Work out the finished part from the listing and answer in its coordinate system (mm). Face numbers are marked on the shaded views. Give positions to 0.01 mm unless a question says otherwise; leave off trailing zeros. Order: outer loops, then holes, each group sorted by start corner. A loop starts at its lowest first (then second) coordinate and runs counter-clockwise, first axis right, second up. Notation, with made-up numbers: M -10.75,78 L 23.25,78 A33 cw 23.25,108 Z; hole C 31,-9.75 d7. An arc over 180 degrees is marked long. One line per item, written item: value.
from build123d import *

# Parameters (mm, degrees)
SKETCH1_W           = 12.7
SKETCH1_H           = 20.193
BOSS_EXTRUDE1_DEPTH = 6.35
SKETCH3_R           = 1.524
CUT_EXTRUDE1_DEPTH  = 25.685415715
SKETCH4_R           = 2.794
CUT_EXTRUDE2_DEPTH  = 0.762
SKETCH8_R           = 1.1938
CUT_EXTRUDE5_DEPTH  = 25.685415715
CUT_EXTRUDE7_DEPTH  = 25.685415715
CUT_EXTRUDE8_DEPTH  = 25.685415715


with BuildPart() as part:
    # Sketch1 → Boss-Extrude1 (new body)
    with BuildSketch(Plane.XY):
        with Locations((6.35, 10.0965)):
            Rectangle(SKETCH1_W, SKETCH1_H)
    extrude(amount=BOSS_EXTRUDE1_DEPTH)

    # Sketch3 → Cut-Extrude1 (cut, through all)
    with BuildSketch(Plane.XY.offset(6.35)):
        with Locations((3.175, 8.509)):
            Circle(SKETCH3_R)
        with Locations((9.525, 8.509)):
            Circle(SKETCH3_R)
    extrude(amount=-CUT_EXTRUDE1_DEPTH, mode=Mode.SUBTRACT)

    # Sketch4 → Cut-Extrude2 (cut)
    with BuildSketch(Plane.XY.offset(6.35)):
        with Locations((3.175, 8.509)):
            Circle(SKETCH4_R)
        with Locations((9.525, 8.509)):
            Circle(SKETCH4_R)
    extrude(amount=-CUT_EXTRUDE2_DEPTH, mode=Mode.SUBTRACT)

    # Sketch8 → Cut-Extrude5 (cut, through all)
    with BuildSketch(Plane(origin=(12.7, 0, 0), x_dir=(0, 0, -1), z_dir=(1, 0, 0))):
        with Locations((-3.175, 17.018)):
            Circle(SKETCH8_R)
    extrude(amount=-CUT_EXTRUDE5_DEPTH, mode=Mode.SUBTRACT)

    # Sketch12 → Cut-Extrude7 (cut, through all)
    with BuildSketch(Plane(origin=(12.7, 0, 0), x_dir=(0, 0, -1), z_dir=(1, 0, 0))):
        with BuildLine():
            Line((-6.35, 20.193), (-3.175, 20.193))
            ThreePointArc((-3.175, 20.193), (-0.92993597, 19.26306403), (0, 17.018))
            Line((0, 17.018), (0, 13.936871151))
            Line((0, 13.936871151), (3.924146207, 13.936871151))
            Line((3.924146207, 13.936871151), (3.924146207, 24.495106429))
            Line((3.924146207, 24.495106429), (-6.35, 24.495106429))
            Line((-6.35, 24.495106429), (-6.35, 20.193))
        make_face()
    extrude(amount=-CUT_EXTRUDE7_DEPTH, mode=Mode.SUBTRACT)

    # Sketch13 → Cut-Extrude8 (cut, through all)
    with BuildSketch(Plane(origin=(12.7, 0, 0), x_dir=(0, 0, -1), z_dir=(1, 0, 0))):
        Polygon((-6.35, 19.431), (8.189826156, 20.193), (-6.35, 20.193), align=None)
    extrude(amount=-CUT_EXTRUDE8_DEPTH, mode=Mode.SUBTRACT)


solid = part.part
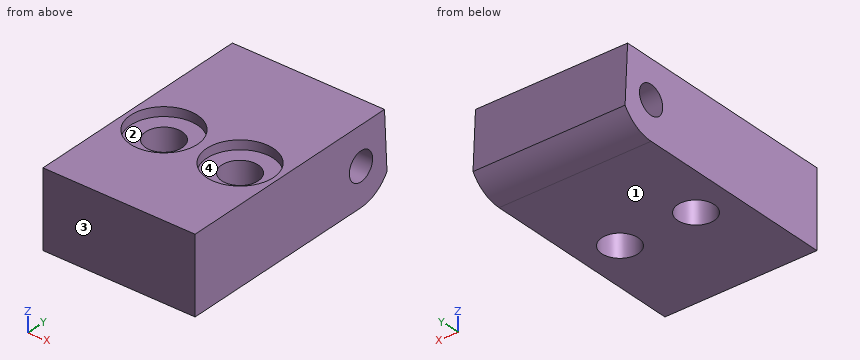
(1) Find the intervals of material crossed by probe 1 along X at (y, z) = (7.25, 4.5); probe 2 along Y at (x, z) = (3.5, 2.5); probe 3 along X at (y, z) = (7.75, 1), in increasing order. Write a range as from..to.
Findings:
probe 1: x = 0..2.32, 4.03..8.67, 10.38..12.7
probe 2: y = 0..7.02, 10..16.03, 18..19.63
probe 3: x = 0..1.85, 4.5..8.2, 10.85..12.7
(2) Section D-D, the plane y = 6.5 is taken. Give the vertices of the cut face in (x, z).
Findings:
outline: M 0,0 L 12.7,0 L 12.7,6.35 L 11.47,6.35 L 11.47,5.59 L 7.58,5.59 L 7.58,6.35 L 5.12,6.35 L 5.12,5.59 L 1.23,5.59 L 1.23,6.35 L 0,6.35 Z
(3) Section B-B, the plane x = 4 is taken. Give the vertices of the cut face in (y, z) (3 decimals).
Findings:
outline: M 0,0 L 7.228,0 L 7.228,5.588 L 5.84,5.588 L 5.84,6.35 L 0,6.35 Z; M 9.79,0 L 17.018,0 A3.175 ccw 19.687,1.456 L 19.431,6.35 L 11.178,6.35 L 11.178,5.588 L 9.79,5.588 Z; hole C 17.018,3.175 d2.388
(4) Section A-A, the plane z = 3 is taken. Give the vertices of the cut face in (x, y) (3 decimals).
Findings:
outline: M 0,0 L 12.7,0 L 12.7,15.837 L 0,15.837 Z; M 0,18.199 L 12.7,18.199 L 12.7,19.607 L 0,19.607 Z; hole C 3.175,8.509 d3.048; hole C 9.525,8.509 d3.048
(5) Determine the mould class of the marked faces 1, 2, 3 and 4 for opening direction Y: pulls with the +Y half, pulls with the -Y half, needs draft (parallel to the pull), parting line crosses it, or undercut.
Findings:
face 1: needs draft
face 2: undercut
face 3: pulls with the -Y half
face 4: undercut
(6) Section C-C, the plane z = 4 is taken. Give the vertices of the cut face in (x, y) (3 decimals).
Findings:
outline: M 0,0 L 12.7,0 L 12.7,16.155 L 0,16.155 Z; M 0,17.881 L 12.7,17.881 L 12.7,19.554 L 0,19.554 Z; hole C 3.175,8.509 d3.048; hole C 9.525,8.509 d3.048
